```python
from build123d import *

# Parameters (mm, degrees)
BOSS_EXTRUDE1_DEPTH                          = 10.32
SKETCH2_R                                    = 12.7
BOSS_EXTRUDE2_DEPTH                          = 6.35
CUT_EXTRUDE3_DEPTH                           = 33.929301541
CUT_EXTRUDE3_DEPTH_BACK                      = 33.929301541
SKETCH9_R                                    = 1.2
CUT_EXTRUDE4_DEPTH                           = 3.175
CBORE_FOR_M6_HEX_SOCKET_HEAD_CAP_SCR_2_COUNT = 2
CBORE_FOR_M6_HEX_SOCKET_HEAD_CAP_SCR_2_PITCH = 38.1
FILLET2_R                                    = 3.175
FILLET3_R                                    = 3.175
CHAMFER2_SIZE                                = 0.8
CHAMFER3_SIZE                                = 0.5


# Some blends are built 0.0001 mm under size
with BuildPart() as part:
    # Sketch1 → Boss-Extrude1 (new body)
    with BuildSketch(Plane(origin=(0, 0, 0), x_dir=(1, 0, 0), z_dir=(0, 1, 0))):
        with BuildLine():
            Line((-12.7, 21.997045256), (-12.7, -21.997045256))
            ThreePointArc((-12.7, -21.997045256), (0, -25.4), (12.7, -21.997045256))
            Line((12.7, -21.997045256), (12.7, 21.997045256))
            ThreePointArc((12.7, 21.997045256), (0, 25.4), (-12.7, 21.997045256))
        make_face()
    extrude(amount=-BOSS_EXTRUDE1_DEPTH)

    # Sketch2 → Boss-Extrude2 (add)
    with BuildSketch(Plane.XZ.offset(10.32)):
        with Locations(Location((0, 0, 0), (0, 0, 180))):
            Circle(SKETCH2_R)
    extrude(amount=BOSS_EXTRUDE2_DEPTH)

    # Sketch9 → Cut-Extrude3 (cut, two sides: drawn at the far end of the back side and taken through both)
    with BuildSketch(Plane.XY.offset(-CUT_EXTRUDE3_DEPTH_BACK)):
        with Locations((1.2, -13.495)):
            Circle(SKETCH9_R)
    extrude(amount=CUT_EXTRUDE3_DEPTH + CUT_EXTRUDE3_DEPTH_BACK, mode=Mode.SUBTRACT)

    # Sketch10 → Cut-Extrude4 (cut, symmetric)
    with BuildSketch(Plane.XY):
        Polygon((9.128125, -16.67), (9.128125, -10.32), (12.7, -10.32), (12.7, 0), (-12.7, 0), (-12.7, -10.32), (-10.326252745, -10.32), (-6.202514528, -16.67), align=None)
    extrude(amount=CUT_EXTRUDE4_DEPTH, both=True, mode=Mode.SUBTRACT)

    # Sketch13 → CBORE for M6 Hex Socket Head Cap Screw2 (revolve, cut)
    with BuildSketch(Plane(origin=(0, 0, -19.05), x_dir=(0, 0, 1), z_dir=(1, 0, 0))):
        Polygon((0, 0), (0, 10.32), (3.5, 10.32), (3.3, 10.12), (3.3, 6.6), (3.5, 6.4), (5.5, 6.4), (5.5, 0.25), (5.75, 0), align=None)
    cbore_for_m6_hex_socket_head_cap_screw2 = revolve(axis=Axis((0, 6.35, -19.05), (0, -1, 0)), mode=Mode.SUBTRACT)

    # CBORE for M6 Hex Socket Head Cap Scr 2: CBORE for M6 Hex Socket Head Cap Screw2 ×2
    with Locations(*[(0, 0, i * CBORE_FOR_M6_HEX_SOCKET_HEAD_CAP_SCR_2_PITCH) for i in range(1, CBORE_FOR_M6_HEX_SOCKET_HEAD_CAP_SCR_2_COUNT)]):
        add(cbore_for_m6_hex_socket_head_cap_screw2, mode=Mode.SUBTRACT)

    # Fillet2
    fillet2_edges = [part.edges().sort_by_distance(p)[0] for p in [
        (9.128125, -13.495, 3.175),
        (9.128125, -13.495, -3.175),
    ]]
    fillet(fillet2_edges, radius=FILLET2_R - 0.0001)  # a hair under: the kernel refuses the full size

    # Fillet3
    fillet3_edges = [part.edges().sort_by_distance(p)[0] for p in [
        (-8.264383637, -13.495, 3.175),
        (-8.264383637, -13.495, -3.175),
    ]]
    fillet(fillet3_edges, radius=FILLET3_R - 0.0001)  # a hair under: the kernel refuses the full size

    # Sketch14 → Cut-Revolve5 (revolve, cut)
    with BuildSketch(Plane.XY, mode=Mode.PRIVATE) as cut_revolve5_sk:
        Polygon((-2.984654144, -12.444678171), (-7.981398467, -15.689601875), (-10.497950031, -14.462197667), (-4.291787828, -10.431868808), align=None)
    revolve(cut_revolve5_sk.sketch.rotate(Axis((-8.485140668, -13.155063983, 0), (-0.8386705679454227, -0.5446390350150291, 0)), 180), axis=Axis((-8.485140668, -13.155063983, 0), (-0.8386705679454227, -0.5446390350150291, 0)), mode=Mode.SUBTRACT)

    # Chamfer2
    chamfer2_edges = [part.edges().sort_by_distance(p)[0] for p in [
        (12.7, -16.67, 0),
    ]]
    chamfer(chamfer2_edges, length=CHAMFER2_SIZE)

    # Chamfer3
    # the kernel refuses this chamfer: 0.5 mm, written as the material it takes off along each edge
    with BuildSketch(Plane(origin=(0, -10.32, 0), x_dir=(-0.5431897052031074, 0, 0.839609995272425), z_dir=(-0.839609995272425, 0, -0.5431897052031074))) as chamfer3_piece_1:
        Polygon((25.4 - CHAMFER3_SIZE, 0), (25.4, CHAMFER3_SIZE), (25.4, 0), align=None)
    revolve(axis=Axis((0, -10.32, 0), (0, 1, 0)), revolution_arc=65.802082053, mode=Mode.SUBTRACT)
    with BuildSketch(Plane(origin=(12.7, -10.32, 23.28288675), x_dir=(-0.9996219169112968, -0.027495876610585647, 0), z_dir=(0, 0, -1)), Plane(origin=(12.7, 0, -1.889158506), x_dir=(0.02749587661058563, -0.9996219169112968, 0), z_dir=(0, 0, -1)), Plane(origin=(12.7, -10.32, -1.889158506), x_dir=(-0.9996219169112968, -0.027495876610585647, 0), z_dir=(0, 0, -1)), Plane(origin=(-12.7, -10.32, 1.889158506), x_dir=(0.9996219169112968, -0.027495876610585647, 0), z_dir=(0, 0, 1)), Plane(origin=(12.7, 0, 23.28288675), x_dir=(0.02749587661058563, -0.9996219169112968, 0), z_dir=(0, 0, -1)), Plane(origin=(-12.7, -10.32, -23.28288675), x_dir=(0.9996219169112968, -0.027495876610585647, 0), z_dir=(0, 0, 1))) as chamfer3_piece_2:
        Polygon((CHAMFER3_SIZE * 0.999621916911, CHAMFER3_SIZE * 0.0274958766106), (-CHAMFER3_SIZE * 0.0274958766106, CHAMFER3_SIZE * 0.999621916911), (0, 0), align=None)
    extrude(amount=21.393728244, mode=Mode.SUBTRACT)
    with BuildSketch(Plane(origin=(-12.7, 0, 1.889158506), x_dir=(0.9996219169112968, 0.02749587661058639, 0), z_dir=(0, 0, 1)), Plane(origin=(-12.7, 0, -23.28288675), x_dir=(0.9996219169112968, 0.02749587661058639, 0), z_dir=(0, 0, 1))) as chamfer3_piece_3:
        Polygon((CHAMFER3_SIZE * 0.999621916911, -CHAMFER3_SIZE * 0.0274958766106), (-CHAMFER3_SIZE * 0.0274958766106, -CHAMFER3_SIZE * 0.999621916911), (0, 0), align=None)
    extrude(amount=21.393728244, mode=Mode.SUBTRACT)
    with BuildSketch(Plane(origin=(13.985841494, 0, 3.175), x_dir=(0, -0.9996219169112968, -0.027495876610586494), z_dir=(-1, 0, 0))) as chamfer3_piece_4:
        Polygon((CHAMFER3_SIZE * 0.999621916911, CHAMFER3_SIZE * 0.0274958766106), (-CHAMFER3_SIZE * 0.0274958766106, CHAMFER3_SIZE * 0.999621916911), (0, 0), align=None)
    extrude(amount=27.971682988, mode=Mode.SUBTRACT)
    with BuildSketch(Plane(origin=(13.985841494, 0, -3.175), x_dir=(0, -0.9996219169112968, 0.027495876610586494), z_dir=(-1, 0, 0))) as chamfer3_piece_5:
        Polygon((CHAMFER3_SIZE * 0.999621916911, -CHAMFER3_SIZE * 0.0274958766106), (-CHAMFER3_SIZE * 0.0274958766106, -CHAMFER3_SIZE * 0.999621916911), (0, 0), align=None)
    extrude(amount=27.971682988, mode=Mode.SUBTRACT)
    with BuildSketch(Plane(origin=(0, -10.32, 0), x_dir=(0.5431897052031078, 0, -0.8396099952724246), z_dir=(0.8396099952724246, 0, 0.5431897052031078))) as chamfer3_piece_6:
        Polygon((25.4 - CHAMFER3_SIZE, 0), (25.4, CHAMFER3_SIZE), (25.4, 0), align=None)
    revolve(axis=Axis((0, -10.32, 0), (0, 1, 0)), revolution_arc=65.802082053, mode=Mode.SUBTRACT)
    with BuildSketch(Plane(origin=(0, 0, 0), x_dir=(-0.5431897052031074, 0, 0.839609995272425), z_dir=(-0.839609995272425, 0, -0.5431897052031074))) as chamfer3_piece_7:
        Polygon((25.4 - CHAMFER3_SIZE, 0), (25.4, -CHAMFER3_SIZE), (25.4, 0), align=None)
    revolve(axis=Axis((0, 0, 0), (0, 1, 0)), revolution_arc=65.802082053, mode=Mode.SUBTRACT)
    with BuildSketch(Plane(origin=(0, 0, 0), x_dir=(0.5431897052031078, 0, -0.8396099952724246), z_dir=(0.8396099952724246, 0, 0.5431897052031078))) as chamfer3_piece_8:
        Polygon((25.4 - CHAMFER3_SIZE, 0), (25.4, -CHAMFER3_SIZE), (25.4, 0), align=None)
    revolve(axis=Axis((0, 0, 0), (0, 1, 0)), revolution_arc=65.802082053, mode=Mode.SUBTRACT)


solid = part.part
```
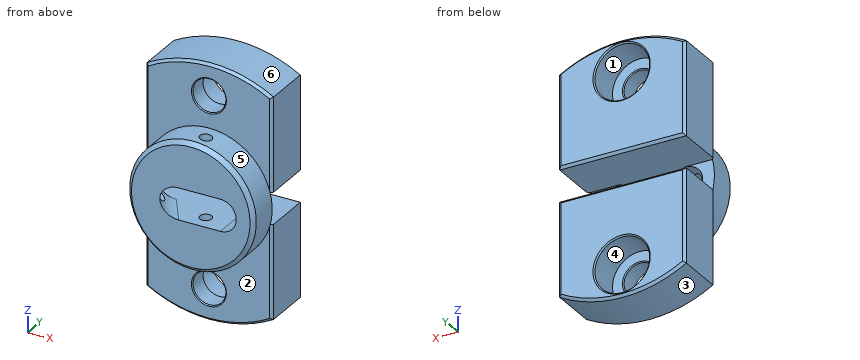
Build history of the part. All positions in model axes, mm. Face numbers are marked on the shaded views. A direction names the side the tool comes from. Round coordinates to 2 decimals unless told otherwise and drop trailing zeros. Write each loop counter-clockwise with the first axis right and the second up, starting at its lowest first coordinate (ties: lowest second). Pieces come first, ordered by that corner, then holes. Notation, with made-up numbers: (23.25, -27.5) -> (35.25, -27.5) arc R26 cw to (35.25, 6.5) -> close; hole circle Ø11 at (-25, -6). An arc over 180 degrees is marked (long way). Put each result on its own line as item: value.
Item 1: Slice it at C-C, the plane y = -3. Give the cut face in (x, z) (3 decimals), plus the area to 3 significant figures.
Here are the results:
outline: (-12.7, -21.997) arc R25.4 ccw to (12.7, -21.997) -> (12.7, -3.175) -> (-12.7, -3.175) -> close; (-12.7, 3.175) -> (12.7, 3.175) -> (12.7, 21.997) arc R25.4 ccw to (-12.7, 21.997) -> close; hole circle Ø11 at (0, -19.05); hole circle Ø11 at (0, 19.05)
area: 883 mm^2
Item 2: Slice it at A-A, the plane y = -7.25. Give the cut face in (x, z) (3 decimals).
Here are the results:
outline: (-12.7, -21.997) arc R25.4 ccw to (12.7, -21.997) -> (12.7, -3.175) -> (-12.7, -3.175) -> close; (-12.7, 3.175) -> (12.7, 3.175) -> (12.7, 21.997) arc R25.4 ccw to (-12.7, 21.997) -> close; hole circle Ø6.6 at (0, -19.05); hole circle Ø6.6 at (0, 19.05)
Item 3: Tool access for the marked faces 4, 5 and 6: list every direction of +Z, -Z, +X, -X, +Y, -Y with a clear straight run to the whole face (end or side of a thin tool).
Here are the results:
face 4: +Y
face 5: -Y
face 6: +Z, +Y, -Y
Item 4: Two-plate mould, pull along Z, no slides. Class the marked faces 1, 2 and 3: pulls with the +Z half, pulls with the -Z half, needs draft (parallel to the pull), parting line crosses it, or undercut.
Here are the results:
face 1: undercut
face 2: needs draft
face 3: pulls with the -Z half
Item 5: Wall check: probe 1 along Z at (x, y) = (0, -3.5) (3 decimals); probe 2 along Z at (x, y) = (0, -7.4) (3 decimals); probe 3 along Y at (x, z) = (1.2, 5.5) (3 decimals). Give the ranges that are in metal, low to high. Write a range as from..to.
Here are the results:
probe 1: z = -25.4..-24.55, -13.55..-3.175, 3.175..13.55, 24.55..25.4
probe 2: z = -25.4..-22.35, -15.75..-3.175, 3.175..15.75, 22.35..25.4
probe 3: y = -16.67..-14.695, -12.295..0
Item 6: Slice it at D-D, the plane x = 1.2. Count the separate pieces of the cut face and the enclosed holes in it, plus the area to 3 significant figures.
Here are the results:
separate pieces: 6
enclosed holes: 0
area: 346 mm^2
Item 7: Slice it at B-B, the plane z = 19.05. Give the cut face in (x, y).
Here are the results:
outline: (-12.7, -9.82) -> (-12.2, -10.32) -> (-3.5, -10.32) -> (-3.3, -10.12) -> (-3.3, -6.6) -> (-3.5, -6.4) -> (-5.5, -6.4) -> (-5.5, -0.25) -> (-5.75, 0) -> (-12.2, 0) -> (-12.7, -0.5) -> close; (3.3, -10.12) -> (3.5, -10.32) -> (12.2, -10.32) -> (12.7, -9.82) -> (12.7, -0.5) -> (12.2, 0) -> (5.75, 0) -> (5.5, -0.25) -> (5.5, -6.4) -> (3.5, -6.4) -> (3.3, -6.6) -> close
Item 8: Flat gauge pins, fed straight in: P1, Ø2, axis at y = -14, z = 11, coming from the +X side; P2, Ø2, axis at x = 1.2, y = -13.495, coming from the +Z side; P3, Ø10, axis at x = 4, z = -17, coming from the -Y side; P4, Ø3.5, axis at x = 9.5, z = -0.5, coming from the +Y side. Where does each tip first touch, or does it go through?
Here are the results:
P1: stops at x = 7.83
P2: passes through
P3: stops at y = -16.11
P4: stops at y = -10.32
